from build123d import *

# Parameters (mm, degrees)
SKETCH1_R           = 10
BOSS_EXTRUDE1_DEPTH = 20
BOSS_EXTRUDE2_DEPTH = 10
BOSS_EXTRUDE3_DEPTH = 10


with BuildPart() as part:
    # Sketch1 → Boss-Extrude1 (new body)
    with BuildSketch(Plane(origin=(0, 0, 0), x_dir=(1, 0, 0), z_dir=(0, 1, 0))):
        with BuildLine():
            Line((-30, 31.581015912), (20, 31.581015912))
            Line((20, 31.581015912), (20, -8.418984088))
            ThreePointArc((20, -8.418984088), (17.071067812, -15.4900519), (10, -18.418984088))
            Line((10, -18.418984088), (-30, -18.418984088))
            Line((-30, -18.418984088), (-30, 31.581015912))
        make_face()
        with Locations(Location((0, 0, 0), (0, 0, 270))):
            Circle(SKETCH1_R, mode=Mode.SUBTRACT)
    extrude(amount=BOSS_EXTRUDE1_DEPTH)

    # Sketch2 → Boss-Extrude2 (add)
    with BuildSketch(Plane.ZY.offset(30)):
        Polygon((18.418984088, 20), (-21.581015912, 20), (-21.581015912, 40), align=None)
    extrude(amount=-BOSS_EXTRUDE2_DEPTH)

    # Sketch3 → Boss-Extrude3 (add)
    with BuildSketch(Plane(origin=(0, 0, -31.581015912), x_dir=(-1, 0, 0), z_dir=(0, 0, -1))):
        Polygon((30, 20), (30, 40), (10, 40), (10, 30), (-10, 30), (-10, 20), align=None)
    extrude(amount=-BOSS_EXTRUDE3_DEPTH)


solid = part.part
Can you work these out from the model? Positions are in its coordinate system, mm. A direction names the side the tool comes from. Give positions to 0.01 mm unless a question says otherwise; leave off trailing zeros. Order: outer loops, then holes, each group sorted by start corner. A loop starts at its lowest first (then second) coordinate and runs counter-clockwise, first axis right, second up. Notation, with made-up numbers: (7.5, -38) - (27.5, -38) arc R24 ccw to (27.5, -18) - close; hole circle Ø9 at (30.25, 71). An arc over 180 degrees is marked (long way). Write each question's results on one line, items separated by ' | '.
1) Suppose I cut it at A-A, the plane x = 0. Write out the boundary of the cut face in (y, z).
Final values:
outline: (0, -31.58) - (30, -31.58) - (30, -21.58) - (20, -21.58) - (20, -10) - (0, -10) - close; (0, 10) - (20, 10) - (20, 18.42) - (0, 18.42) - close
2) Suppose I cut it at D-D, the plane y = 5. Write out the boundary of the cut face in (x, z).
Final values:
outline: (-30, -31.58) - (20, -31.58) - (20, 8.42) arc R10 ccw to (10, 18.42) - (-30, 18.42) - close; hole circle Ø20 at (0, 0)
3) Please list where these lines run through material, in increasing order: line 1 along X through (y, z) = (7, 0); line 2 along Y through (x, z) = (-18, -16); line 3 along X through (y, z) = (35, -23). Write a range as [from, to].
Final values:
line 1: x = [-30, -10], [10, 20] | line 2: y = [0, 20] | line 3: x = [-30, -10]
4) Suppose I cut it at B-B, the plane z = -3.5. Write out the boundary of the cut face in (x, y).
Final values:
outline: (-30, 0) - (-9.37, 0) - (-9.37, 20) - (-20, 20) - (-20, 30.96) - (-30, 30.96) - close; (9.37, 0) - (20, 0) - (20, 20) - (9.37, 20) - close
5) On a 3-axis mill with a long thin cutter (end or side, diameter ignored), from which of +Z, -Z, +X, -X, +Y, -Y can I reach the whole of each face in a straight line? I mean faces 1 (the face through (-8, 28, -21.581)), 2 (the face through (10, 25, -27)), 3 (the face through (-9.76, 9.86, -2.17)). Say none if no direction works.
Final values:
face 1: +Z, +X, +Y | face 2: +Z, -Z, +X, +Y | face 3: +Y, -Y
6) Suppose I cut it at C-C, the plane z = -27.5. Write out the boundary of the cut face in (x, y), then the cut area to 3 significant figures.
Final values:
outline: (-30, 0) - (20, 0) - (20, 20) - (10, 20) - (10, 30) - (-10, 30) - (-10, 40) - (-30, 40) - close | area: 1,600 mm^2
7) I'm going to push flat-ended pins straight in: pin 1 Ø3 at (y, z) = (24.5, -25) entering from +X; pin 2 Ø1 at (x, y) = (-3.5, 28.5) entering from +Z; pin 3 Ø6 at (y, z) = (33, -2) entering from +X. Where does each tip first touch, or does it pass through?
Final values:
pin 1: stops at x = 10 | pin 2: stops at z = -21.58 | pin 3: stops at x = -20
